from build123d import *

# Parameters (mm, degrees)
SKETCH1_R               = 2.8
SKETCH1_W               = 55.97
SKETCH1_H               = 4
SKETCH1_W_2             = 2
BOSS_EXTRUDE1_DEPTH     = 6
SKETCH2_R               = 2.8
BOSS_EXTRUDE2_DEPTH     = 3.5
SKETCH3_R               = 1.6
CUT_EXTRUDE1_DEPTH      = 10
SKETCH4_R               = 3
CUT_EXTRUDE2_DEPTH      = 28.03
BOSS_EXTRUDE3_DEPTH     = 20.015
SKETCH6_R               = 2
CUT_EXTRUDE3_DEPTH      = 6
CUT_EXTRUDE6_DEPTH      = 53.87032367
CUT_EXTRUDE6_DEPTH_BACK = 8
SKETCH10_R              = 2


with BuildPart() as part:
    # Sketch1 → Boss-Extrude1 (new, symmetric)
    # profile 1 of 8: a face of its own
    with BuildSketch(Plane(origin=(0, 0, 0), x_dir=(1, 0, 0), z_dir=(0, 1, 0))):
        with BuildLine():
            ThreePointArc((24, -0.115), (21.182179477, -1.282179477), (20.015, -4.1))
            Line((20.015, -4.1), (20.015, -10.015))
            Line((20.015, -10.015), (-20.015, -10.015))
            Line((-20.015, -10.015), (-20.015, 10.015))
            Line((-20.015, 10.015), (20.015, 10.015))
            Line((20.015, 10.015), (20.015, 4.1))
            ThreePointArc((20.015, 4.1), (21.182179477, 1.282179477), (24, 0.115))
            ThreePointArc((24, 0.115), (26.817820523, 1.282179477), (27.985, 4.1))
            Line((27.985, 4.1), (27.985, 14.015))
            Line((27.985, 14.015), (-27.985, 14.015))
            Line((-27.985, 14.015), (-27.985, -14.015))
            Line((-27.985, -14.015), (27.985, -14.015))
            Line((27.985, -14.015), (27.985, -4.1))
            ThreePointArc((27.985, -4.1), (26.817820523, -1.282179477), (24, -0.115))
        make_face()
        with Locations(Location((-24, -5, 0), (0, 0, 270))):
            Circle(SKETCH1_R, mode=Mode.SUBTRACT)
        with Locations(Location((-24, 5, 0), (0, 0, 270))):
            Circle(SKETCH1_R, mode=Mode.SUBTRACT)
        with Locations(Location((24, -5, 0), (0, 0, 270))):
            Circle(SKETCH1_R, mode=Mode.SUBTRACT)
        with Locations(Location((24, 5, 0), (0, 0, 270))):
            Circle(SKETCH1_R, mode=Mode.SUBTRACT)
    # profile 2 of 8: a face of its own
    with BuildSketch(Plane(origin=(0, 0, 0), x_dir=(1, 0, 0), z_dir=(0, 1, 0))):
        with Locations((0, -16.015)):
            Rectangle(SKETCH1_W, SKETCH1_H)
    # profile 3 of 8: a face of its own
    with BuildSketch(Plane(origin=(0, 0, 0), x_dir=(1, 0, 0), z_dir=(0, 1, 0))):
        Polygon((27.985, 4.1), (27.985, 0.115), (29.985, 0.115), (29.985, 14.015), (27.985, 14.015), align=None)
    # profile 4 of 8: a face of its own
    with BuildSketch(Plane(origin=(0, 0, 0), x_dir=(1, 0, 0), z_dir=(0, 1, 0))):
        Polygon((29.985, -0.115), (27.985, -0.115), (27.985, -4.1), (27.985, -14.015), (29.985, -14.015), align=None)
    # profile 5 of 8: a face of its own
    with BuildSketch(Plane(origin=(0, 0, 0), x_dir=(1, 0, 0), z_dir=(0, 1, 0))):
        with BuildLine():
            Line((27.985, -4.1), (27.985, -0.115))
            Line((27.985, -0.115), (24, -0.115))
            ThreePointArc((24, -0.115), (26.817820523, -1.282179477), (27.985, -4.1))
        make_face()
    # profile 6 of 8: a face of its own
    with BuildSketch(Plane(origin=(0, 0, 0), x_dir=(1, 0, 0), z_dir=(0, 1, 0))):
        with BuildLine():
            Line((24, 0.115), (27.985, 0.115))
            Line((27.985, 0.115), (27.985, 4.1))
            ThreePointArc((27.985, 4.1), (26.817820523, 1.282179477), (24, 0.115))
        make_face()
    # profile 7 of 8: a face of its own
    with BuildSketch(Plane(origin=(0, 0, 0), x_dir=(1, 0, 0), z_dir=(0, 1, 0))):
        with Locations((28.985, -16.015)):
            Rectangle(SKETCH1_W_2, SKETCH1_H)
    # profile 8 of 8: a face of its own
    with BuildSketch(Plane(origin=(0, 0, 0), x_dir=(1, 0, 0), z_dir=(0, 1, 0))):
        Polygon((-29.985, 14.015), (-29.985, -18.015), (-27.985, -18.015), (-27.985, -14.015), (-27.985, 14.015), align=None)
    extrude(amount=BOSS_EXTRUDE1_DEPTH, both=True)

    # Sketch2 → Boss-Extrude2 (add)
    with BuildSketch(Plane.XZ.offset(6)):
        with Locations(Location((24, -5, 0), (0, 0, 90))):
            Circle(SKETCH2_R)
        with Locations(Location((24, 5, 0), (0, 0, 90))):
            Circle(SKETCH2_R)
        with Locations(Location((-24, -5, 0), (0, 0, 90))):
            Circle(SKETCH2_R)
        with Locations(Location((-24, 5, 0), (0, 0, 90))):
            Circle(SKETCH2_R)
    extrude(amount=-BOSS_EXTRUDE2_DEPTH)

    # Sketch3 → Cut-Extrude1 (cut)
    with BuildSketch(Plane.XY.offset(18.015)):
        with Locations((10.015, 0)):
            Circle(SKETCH3_R)
    extrude(amount=-CUT_EXTRUDE1_DEPTH, mode=Mode.SUBTRACT)

    # Sketch4 → Cut-Extrude2 (cut)
    with BuildSketch(Plane(origin=(0, 0, -14.015), x_dir=(-1, 0, 0), z_dir=(0, 0, -1))):
        with Locations((-10.015, 0)):
            Circle(SKETCH4_R)
    extrude(amount=-CUT_EXTRUDE2_DEPTH, mode=Mode.SUBTRACT)

    # Sketch5 → Boss-Extrude3 (add)
    with BuildSketch(Plane(origin=(0, 0, 0), x_dir=(0, 0, -1), z_dir=(1, 0, 0))):
        Polygon((-18.015, -6), (-10.015, -6), (-10.015, -21.5), (6.985, -21.5), (6.985, -29.5), (-18.015, -29.5), align=None)
    extrude(amount=BOSS_EXTRUDE3_DEPTH)

    # Sketch6 → Cut-Extrude3 (cut)
    with BuildSketch(Plane.XZ.offset(29.5)):
        with Locations(Location((10.015, 0, 0), (0, 0, 270))):
            Circle(SKETCH6_R)
    extrude(amount=-CUT_EXTRUDE3_DEPTH, mode=Mode.SUBTRACT)

    # Sketch10 → Cut-Extrude6 (cut, two sides: drawn at the far end of the back side and taken through both)
    with BuildSketch(Plane.XY.offset(18.015).offset(-CUT_EXTRUDE6_DEPTH_BACK)):
        with Locations(Location((-14.485, 0, 0), (0, 0, 180))):
            Circle(SKETCH10_R)
    extrude(amount=CUT_EXTRUDE6_DEPTH + CUT_EXTRUDE6_DEPTH_BACK, mode=Mode.SUBTRACT)


solid = part.part
Check sheet for the modelled part. Datum: model origin and axes. Units: mm. A direction names the side the tool comes from. Give positions to 0.01 mm unless a question says otherwise; leave off trailing zeros. Order: outer loops, then holes, each group sorted by start corner. A loop starts at its lowest first (then second) coordinate and runs counter-clockwise, first axis right, second up. Notation, with made-up numbers: (-33, -37.75) - (-25, -37.75) arc R32 ccw to (-25, -7.75) - close; hole circle Ø3 at (8.25, 26). An arc over 180 degrees is marked (long way). Answer as CSV lines item,"result".
1. Section check A-A (z = -9). Record the boundary of the cut face in (x, y) (3 decimals).
Result sheet:
outline,"(-29.985, -6) - (-20.015, -6) - (-20.015, 6) - (-29.985, 6) - close; (20.015, -6) - (29.985, -6) - (29.985, 6) - (20.015, 6) - close"
2. Section check C-C (y = 0). State how many separate pieces and enclosed holes the cut face has, then the cut area to 3 significant figures.
Result sheet:
separate pieces,"4"
enclosed holes,"4"
area,"919 mm²"
3. Go/stop test with flat-tipped pins: P1, Ø10, axis at y = -18, z = -7, coming from the +X side (3 decimals); P2, Ø3, axis at x = -25, z = -5, coming from the +Y side; P3, Ø1.8, axis at x = 9.5, y = 0, coming from the -Z side; P4, Ø2.5, axis at x = -14.485, y = 0, coming from the +Z side (3 decimals). Record where each tip stops, or that it passes through.
Result sheet:
P1,"x = 20.015"
P2,"y = -2.5"
P3,"through"
P4,"z = -10.015"
4. Mould release check, pull along Z, two halves, no side actions. Record for faces 1 (the face through (21.151, 0.084, -1.313)), 2 (the face through (-20.4, -6, 1.8)), 3 (the face through (-21.64, 1.69, 6.51)): released by +Z, released by -Z, zero draft, split by the parting line, or undercut.
Result sheet:
face 1,"undercut"
face 2,"zero draft"
face 3,"undercut"
5. Tool access check on faces 4 (the face through (27, 0, 0.115)), 5 (the face through (20.015, 0, 7)), 6 (the face through (10, -23.5, 0)), 7 (the face through (0, -23, 8)), 8 (the face through (12.396, -1.825, 11.987)). Record the directions out of +Z, -Z, +X, -X, +Y, -Y that give a thin tool (end or side, any length) a straight path to the whole face; none if there is none.
Result sheet:
face 4,"+X, +Y, -Y"
face 5,"+Y"
face 6,"-Y"
face 7,"+Z, -Z, -X, -Y"
face 8,"-Z"
6. Scan lines: probe 1 along X at (y, z) = (1.25, 5) (3 decimals); probe 2 along Z at (x, y) = (24, 1) (3 decimals); probe 3 along Z at (x, y) = (-24, 2) (3 decimals). Record each from-to range of solid material in increasing order. Write a range as from..to.
Result sheet:
probe 1,"-29.985..-26.8, -21.2..-20.015, 20.015..21.2, 26.8..29.985"
probe 2,"-14.015..-7.8, -2.2..-0.115, 0.115..2.2, 7.8..18.015"
probe 3,"-14.015..-7.8, -2.2..2.2, 7.8..18.015"
7. Section check D-D (z = -5). Record the boundary of the cut face in (x, y) (3 decimals).
Result sheet:
outline,"(-29.985, -6) - (-20.015, -6) - (-20.015, 6) - (-21.2, 6) - (-21.2, -2.5) - (-26.8, -2.5) - (-26.8, 6) - (-29.985, 6) - close; (0, -29.5) - (20.015, -29.5) - (20.015, -21.5) - (0, -21.5) - close; (20.015, -6) - (29.985, -6) - (29.985, 6) - (26.8, 6) - (26.8, -2.5) - (21.2, -2.5) - (21.2, 6) - (20.015, 6) - close"
8. Section check B-B (x = -11). Record the boundary of the cut face in (y, z) (3 decimals), then the cut area to 3 significant figures.
Result sheet:
outline,"(-6, -14.015) - (6, -14.015) - (6, -10.015) - (-6, -10.015) - close; (-6, 10.015) - (6, 10.015) - (6, 18.015) - (-6, 18.015) - close"
area,"144 mm²"
